from build123d import *

# Parameters (mm, degrees)
SKETCH_1_W      = 50
SKETCH_1_H      = 8
EXTRUDE_1_DEPTH = 40


with BuildPart() as part:
    # 扫描1: sweep along a path in 草图2
    with BuildLine(Plane(origin=(0, 0, 0), x_dir=(0, 0, -1), z_dir=(1, 0, 0))) as sweep_1_path:
        Line((0, 55.298323556), (-160, 55.298323556))
    # 草图1 → 扫描1 (sweep)
    with BuildSketch(Plane.XY):
        Rectangle(SKETCH_1_W, SKETCH_1_H)
    sweep(path=sweep_1_path.line)

    # 草图4 → 凸台-拉伸1 (add)
    with BuildSketch(Plane.XY.offset(160)):
        with BuildLine():
            Line((-50, -25), (-25, 4))
            Line((-25, 4), (25, 4))
            Line((25, 4), (50, -25))
            Line((50, -25), (50, -75))
            Line((50, -75), (42, -75))
            Line((42, -75), (42, -31.238336961))
            ThreePointArc((42, -31.238336961), (0, -4), (-42, -31.238336961))
            Line((-42, -31.238336961), (-42, -75))
            Line((-42, -75), (-50, -75))
            Line((-50, -75), (-50, -25))
        make_face()
    extrude(amount=-EXTRUDE_1_DEPTH)


solid = part.part
Work out the finished part from the listing and answer in its coordinate system (mm). A direction names the side the tool comes from. Coordinates: 2 decimals unless noted, no trailing zeros. Loops run counter-clockwise (first coordinate to the right, second up) from the corner with the lowest first, then second, coordinate; pieces in that order, holes last. Notation, with made-up numbers: M 37,77.5 L 80,77.5 A24 ccw 80,88.5 Z; hole C 72,47.5 d1. An arc over 180 degrees is marked long. Answer in a Markdown table with one row per item. Add a question column.
1. Find section B-B, the plane x = 17. Write down the section's boundary in (y, z), then the cut area to 3 significant figures.
2. Flat-ended cylindrical pins translate along their axes: P1, Ø10, axis at y = -5.5, z = 16, coming from the +X side; P2, Ø2.5, axis at y = -0.5, z = 72, coming from the -X side; P3, Ø25, axis at x = -25, y = -24, coming from the -Z side. Find the tip coordinate at first contact, or state that the pin passes through.
3. The mould has two halves that part along X. Classify faces 1 (the cylindrical face through (0.741, -4.006, 140.28)), 2 (the flat face through (-25, 0, 61)), 3 (the flat face through (0, 0, 0)), 4 (the flat face through (-42, -53, 140)): pulls with the +X half, pulls with the -X half, needs draft (parallel to the pull), parting line crosses it, or undercut.
4. Find section C-C, the plane y = -2. Write down the section's boundary in (x, z).
5. Consider L1, parallel to X at y = -44, z = 120.5; L2, parallel to Y at x = 23, z = 25.5; L3, parallel to Z at x = -42.5, y = -62. Determine where each line is inside the solid, lowest interval first.
6. A tool of negligible diameter and unlimited length cuts with its end or side. For faces 5 (the flat face through (42, -53, 140)), 6 (the flat face through (-37.67, -10.7, 140.28)), 7 (the flat face through (0, -4, 61)), 8 (the flat face through (25, 0, 61)), from which of +Z, -Z, +X, -X, +Y, -Y can it reach the whole face along a straight path? Write none if from no direction.
7. Find section D-D, the plane y = -27.5. Write down the section's boundary in (x, z).
8. Find section A-A, the plane y = -49. Write down the section's boundary in (x, z).
Reported:
| question | item | result |
|---|---|---|
| 1 | outline | M -7.26,120 L -4,120 L -4,0 L 4,0 L 4,160 L -7.26,160 Z |
| 1 | area | 1,410 mm^2 |
| 2 | P1 | stops at x = 25 |
| 2 | P2 | stops at x = -25 |
| 2 | P3 | stops at z = 120 |
| 3 | face 1 | undercut |
| 3 | face 2 | pulls with the -X half |
| 3 | face 3 | needs draft |
| 3 | face 4 | undercut |
| 4 | outline | M -30.17,120 L -25,120 L -25,0 L 25,0 L 25,120 L 30.17,120 L 30.17,160 L -30.17,160 Z |
| 5 | L1 | x = -50 to -42, 42 to 50 |
| 5 | L2 | y = -4 to 4 |
| 5 | L3 | z = 120 to 160 |
| 6 | face 5 | +Z, -Z, -Y |
| 6 | face 6 | +Z, -Z, -X, +Y |
| 6 | face 7 | -Z, +X, -X, -Y |
| 6 | face 8 | -Z, +X, +Y, -Y |
| 7 | outline | M -50,120 L -40.12,120 L -40.12,160 L -50,160 Z; M 40.12,120 L 50,120 L 50,160 L 40.12,160 Z |
| 8 | outline | M -50,120 L -42,120 L -42,160 L -50,160 Z; M 42,120 L 50,120 L 50,160 L 42,160 Z |
